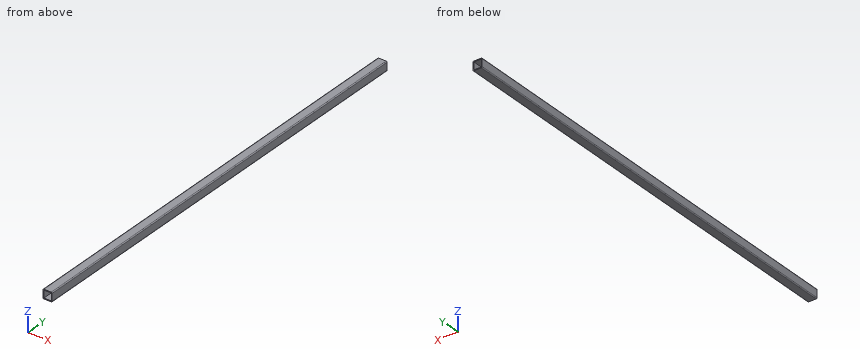
```python
from build123d import *

# Parameters (mm, degrees)
SKETCH4_W           = 25.4
SKETCH4_H           = 25.4
BOSS_EXTRUDE6_DEPTH = 1219.2
SHELL1_T            = -2.54
FILLET1_R           = 2.54


with BuildPart() as part:
    # Sketch4 → Boss-Extrude6 (new body)
    with BuildSketch(Plane(origin=(0, 0, 0), x_dir=(1, 0, 0), z_dir=(0, 1, 0))):
        Rectangle(SKETCH4_W, SKETCH4_H)
    extrude(amount=BOSS_EXTRUDE6_DEPTH)

    # Shell1
    shell1_openings = [part.faces().sort_by_distance(p)[0] for p in [
        (0, 1219.2, 0),
        (0, 0, 0),
    ]]
    offset(amount=SHELL1_T, openings=shell1_openings, kind=Kind.INTERSECTION)

    # Fillet1
    fillet1_edges = [part.edges().sort_by_distance(p)[0] for p in [
        (12.7, 609.6, -12.7),
        (12.7, 609.6, 12.7),
        (-12.7, 609.6, 12.7),
        (-12.7, 609.6, -12.7),
    ]]
    fillet(fillet1_edges, radius=FILLET1_R)


solid = part.part
```
Geometry: final body of the model. Coordinates: model frame, mm. Coordinates: 2 decimals unless noted, no trailing zeros. Order: outer loops, then holes, each group sorted by start corner. A loop starts at its lowest first (then second) coordinate and runs counter-clockwise, first axis right, second up. Notation, with made-up numbers: (24, 39) -> (52, 39) arc R22 ccw to (52, 52) -> close; hole circle Ø6 at (-1.75, 68). An arc over 180 degrees is marked (long way). Answer in a Markdown table with one row per item.
Item 1: Section A-A on z = -1.25. Output: boundary loops of the cut face in (x, y).
Return value:
| item | result |
|---|---|
| outline | (-12.7, 0) -> (-10.16, 0) -> (-10.16, 1219.2) -> (-12.7, 1219.2) -> close; (10.16, 0) -> (12.7, 0) -> (12.7, 1219.2) -> (10.16, 1219.2) -> close |
Item 2: Section C-C on x = 0.75. Output: boundary loops of the cut face in (y, z), plus the area to 3 significant figures.
Return value:
| item | result |
|---|---|
| outline | (0, -12.7) -> (1219.2, -12.7) -> (1219.2, -10.16) -> (0, -10.16) -> close; (0, 10.16) -> (1219.2, 10.16) -> (1219.2, 12.7) -> (0, 12.7) -> close |
| area | 6,190 mm² |
Item 3: Ray query, L1, parallel to Z at x = 1, y = 1024; L2, parallel to X at y = 78, z = -10.75. Return the intervals inside material, ascending.
Return value:
| item | result |
|---|---|
| L1 | z = -12.7 to -10.16, 10.16 to 12.7 |
| L2 | x = -12.63 to 12.63 |
Item 4: Section B-B on y = 76. Output: boundary loops of the cut face in (x, z), plus the area to 3 significant figures.
Return value:
| item | result |
|---|---|
| outline | (-12.7, -10.16) arc R2.54 ccw to (-10.16, -12.7) -> (10.16, -12.7) arc R2.54 ccw to (12.7, -10.16) -> (12.7, 10.16) arc R2.54 ccw to (10.16, 12.7) -> (-10.16, 12.7) arc R2.54 ccw to (-12.7, 10.16) -> close; hole (-10.16, -10.16) -> (10.16, -10.16) -> (10.16, 10.16) -> (-10.16, 10.16) -> close |
| area | 227 mm² |
